CAD build for the part. Positions are in the model's coordinates, mm. Face numbers are marked on the shaded views. Give positions to 0.01 mm unless a question says otherwise; leave off trailing zeros. Loops run counter-clockwise (first coordinate to the right, second up) from the corner with the lowest first, then second, coordinate; pieces in that order, holes last. Notation, with made-up numbers: (68, 83.25) -> (94, 83.25) arc R19 ccw to (94, 113.25) -> close; hole circle Ø10 at (-40, 57). An arc over 180 degrees is marked (long way). Use one line per item in the form item = value.
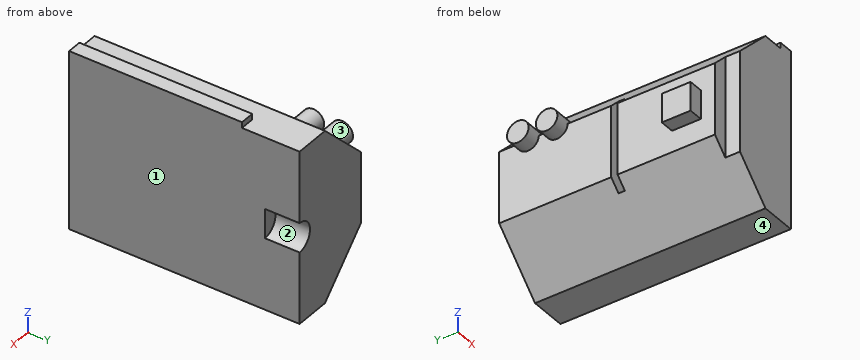
```python
from build123d import *

# Parameters (mm, degrees)
BOSS_EXTRUDE1_DEPTH      = 80
CUT_EXTRUDE1_DEPTH       = 1.1
SKETCH4_W                = 30
SKETCH4_H                = 60
CUT_EXTRUDE2_DEPTH       = 91.553851381
SKETCH5_R                = 5.1
CUT_EXTRUDE3_DEPTH       = 12
BOSS_EXTRUDE2_DEPTH      = 5
BOSS_EXTRUDE2_DEPTH_BACK = 12
SKETCH6_R                = 3.75
SKETCH6_W                = 10
SKETCH6_H                = 10
SKETCH7_W                = 5
SKETCH7_H                = 60
BOSS_EXTRUDE3_DEPTH      = 2
SKETCH8_W                = 5.1
SKETCH8_H                = 5.1
CUT_EXTRUDE4_DEPTH       = 106.948100502


with BuildPart() as part:
    # Sketch1 → Boss-Extrude1 (new body)
    with BuildSketch(Plane(origin=(0, 0, 0), x_dir=(1, 0, 0), z_dir=(0, 1, 0))):
        Polygon((12.426406871, -30), (30, -12.426406871), (30, 12.426406871), (12.426406871, 30), (-12.426406871, 30), (-30, 12.426406871), (-30, -12.426406871), (-12.426406871, -30), align=None)
    extrude(amount=BOSS_EXTRUDE1_DEPTH)

    # Sketch3 → Cut-Extrude1 (cut, symmetric)
    with BuildSketch(Plane(origin=(0, 40, 0), x_dir=(1, 0, 0), z_dir=(0, 1, 0))):
        Polygon((40, 25), (10, 5.1), (10, -5.1), (40, -25), align=None)
    cut_extrude1 = extrude(amount=CUT_EXTRUDE1_DEPTH, both=True, mode=Mode.SUBTRACT)

    # Mirror1: Cut-Extrude1 across plane
    add(cut_extrude1.mirror(Plane(origin=(0, 0, 0), x_dir=(0, 0, 1), z_dir=(1, 0, 0))), mode=Mode.SUBTRACT)

    # Sketch4 → Cut-Extrude2 (cut, through all)
    with BuildSketch(Plane(origin=(0, 80, 0), x_dir=(1, 0, 0), z_dir=(0, 1, 0))):
        with Locations((15, 0)):
            Rectangle(SKETCH4_W, SKETCH4_H)
    extrude(amount=-CUT_EXTRUDE2_DEPTH, mode=Mode.SUBTRACT)

    # Sketch5 → Cut-Extrude3 (cut)
    with BuildSketch(Plane(origin=(0, 80, 0), x_dir=(1, 0, 0), z_dir=(0, 1, 0))):
        Circle(SKETCH5_R)
    extrude(amount=-CUT_EXTRUDE3_DEPTH, mode=Mode.SUBTRACT)

    # Sketch6 → Boss-Extrude2 (add, two sides: drawn at the far end of the back side and taken through both)
    with BuildSketch(Plane.ZY.offset(30).offset(-BOSS_EXTRUDE2_DEPTH_BACK)):
        with Locations((12.426406871, 70)):
            Circle(SKETCH6_R)
        with Locations((12.426406871, 60)):
            Circle(SKETCH6_R)
        with Locations((0, 15)):
            Rectangle(SKETCH6_W, SKETCH6_H)
    extrude(amount=BOSS_EXTRUDE2_DEPTH + BOSS_EXTRUDE2_DEPTH_BACK)

    # Sketch7 → Boss-Extrude3 (add)
    with BuildSketch(Plane.XY.offset(30)):
        with Locations((-2.5, 30)):
            Rectangle(SKETCH7_W, SKETCH7_H)
    extrude(amount=BOSS_EXTRUDE3_DEPTH)

    # Sketch8 → Cut-Extrude4 (cut, through all)
    with BuildSketch(Plane.XY.offset(30)):
        with Locations((-27.45, 2.55)):
            Rectangle(SKETCH8_W, SKETCH8_H)
    extrude(amount=-CUT_EXTRUDE4_DEPTH, mode=Mode.SUBTRACT)


solid = part.part
```
1. Drop flat-ended pins along their axis: P1, Ø3.5, axis at x = -7.5, y = 59.5, coming from the +Z side; P2, Ø4, axis at y = 46.5, z = -1, coming from the -X side; P3, Ø1, axis at x = -22, y = 32.5, coming from the -Z side. Give the stop position or say it passes through.
Result sheet:
P1 = 30
P2 = -30
P3 = -20.93
2. Mould opens along Z. For the marked faces 1, 2, 3 and 4 say: pulls with the +Z half, pulls with the -Z half, needs draft (parallel to the pull), parting line crosses it, or undercut.
Result sheet:
face_1 = needs draft
face_2 = undercut
face_3 = parting line crosses it
face_4 = pulls with the -Z half
3. Cut at C-C, the plane z = 0. Write the cut outline in (x, y), then the cut area to 3 significant figures.
Result sheet:
outline = (-35, 10) -> (-30, 10) -> (-30, 5.1) -> (-24.9, 5.1) -> (-24.9, 0) -> (0, 0) -> (0, 68) -> (-5.1, 68) -> (-5.1, 80) -> (-30, 80) -> (-30, 41.1) -> (-10, 41.1) -> (-10, 38.9) -> (-30, 38.9) -> (-30, 20) -> (-35, 20) -> close
area = 2,320 mm^2
4. Cut at A-A, the plane x = -32. Write the cut outline in (y, z), then the cut area to 3 significant figures.
Result sheet:
outline = (10, -5) -> (20, -5) -> (20, 5) -> (10, 5) -> close; circle Ø7.5 at (60, 12.43); circle Ø7.5 at (70, 12.43)
area = 188 mm^2
5. Cut at D-D, the plane x = -28. Write the cut outline in (y, z).
Result sheet:
outline = (5.1, -14.43) -> (38.9, -14.43) -> (38.9, 14.43) -> (5.1, 14.43) -> close; (41.1, -14.43) -> (80, -14.43) -> (80, 14.43) -> (73.17, 14.43) arc R3.75 ccw to (66.83, 14.43) -> (63.17, 14.43) arc R3.75 ccw to (56.83, 14.43) -> (41.1, 14.43) -> close
6. Cut at B-B, the plane y = 70. Write the cut outline in (x, z), then the cut area to 3 significant figures.
Result sheet:
outline = (-35, 8.68) -> (-30, 8.68) -> (-30, -12.43) -> (-12.43, -30) -> (0, -30) -> (0, -5.1) arc R5.1 cw to (0, 5.1) -> (0, 30) -> (-12.43, 30) -> (-26.25, 16.18) -> (-35, 16.18) -> close
area = 1,490 mm^2
7. Drill centre lines: line 1 (Y direction, x = -22, z = -6.5); line 2 (Y direction, x = -28, z = -0.5); line 3 (X direction, y = 39.5, z = 2.5). Where is each one in solid material? Low to high.
Result sheet:
line_1 = 0 to 38.9, 41.1 to 80
line_2 = 5.1 to 38.9, 41.1 to 80
line_3 = -10 to 0
